from build123d import *

# Parameters (mm, degrees)
CROQUIS2_R              = 19
SALIENTE_EXTRUIR1_DEPTH = 7
CROQUIS2_4_R            = 6
SALIENTE_EXTRUIR2_DEPTH = 8
CROQUIS2_5_R            = 2
CORTAR_EXTRUIR2_DEPTH   = 8
CROQUIS5_R              = 3
CORTAR_EXTRUIR3_DEPTH   = 2


with BuildPart() as part:
    # Croquis2 → Saliente-Extruir1 (new body)
    with BuildSketch(Plane(origin=(0, 0, 0), x_dir=(1, 0, 0), z_dir=(0, 1, 0))):
        Circle(CROQUIS2_R)
    extrude(amount=SALIENTE_EXTRUIR1_DEPTH)

    # Croquis2<4> → Saliente-Extruir2 (add)
    with BuildSketch(Plane(origin=(0, 0, 0), x_dir=(1, 0, 0), z_dir=(0, 1, 0))):
        Circle(CROQUIS2_4_R)
    extrude(amount=-SALIENTE_EXTRUIR2_DEPTH)

    # Croquis2<5> → Cortar-Extruir2 (cut, through all)
    with BuildSketch(Plane(origin=(0, 0, 0), x_dir=(1, 0, 0), z_dir=(0, 1, 0))):
        with Locations((-15, 0)):
            Circle(CROQUIS2_5_R)
    extrude(amount=CORTAR_EXTRUIR2_DEPTH, mode=Mode.SUBTRACT)

    # Croquis5 → Cortar-Extruir3 (cut)
    with BuildSketch(Plane(origin=(0, 7, 0), x_dir=(1, 0, 0), z_dir=(0, 1, 0))):
        with Locations((-15, 0)):
            Circle(CROQUIS5_R)
    extrude(amount=-CORTAR_EXTRUIR3_DEPTH, mode=Mode.SUBTRACT)


solid = part.part
Design review of the part built by this model. Coordinates are the model's own, in mm. A direction names the side the tool comes from. Round coordinates to 2 decimals unless told otherwise and drop trailing zeros. Loops run counter-clockwise (first coordinate to the right, second up) from the corner with the lowest first, then second, coordinate; pieces in that order, holes last. Notation, with made-up numbers: (49, 40.5) - (102, 40.5) arc R34 ccw to (102, 77.5) - close; hole circle Ø9 at (68, 76.25). An arc over 180 degrees is marked (long way). One line per item, written item: value. Start each with the question number.
1) Consider section A-A on z = 0. Give the boundary of the cut face in (x, y), then the cut area to 3 significant figures.
2) To check wall thickness, follow L1, parallel to X at y = 2.15, z = 0; L2, parallel to X at y = 5.7, z = 0; L3, parallel to Y at x = 17, z = 6. State the ranges of each line that lie inside material, in increasing order. Write a range as from..to.
3) Consider section C-C on x = -15. Give the boundary of the cut face in (y, z), then the cut area to 3 significant figures.
4) Insertion check: pin 1 Ø4 at (x, z) = (-15, 14) entering from +Y; pin 2 Ø1.5 at (x, y) = (-13, 5) entering from -Z; pin 3 Ø8 at (x, y) = (3, -6.5) entering from -Z; pin 4 Ø4 at (y, z) = (2, 4) entering from +X. Each pin has a flat end and moves straight along its axis. Give the tip position at first contact, or say it passes through.
5) Consider section D-D on y = 3.5. Give the boundary of the cut face in (x, z), then the cut area to 3 significant figures.
6) Consider section B-B on x = 0. Give the boundary of the cut face in (y, z), then the cut area to 3 significant figures.
7) Draft analysis for pull direction X (two halves, no side actions). For faces 4 (the cylindrical face through (-18, 6, 0)), 5 (the cylindrical face through (8.767, 3.451, 16.856)), 6 (the flat face through (-4.5, 0, -4.5)), state which applies: +X half, -X half, draft (parallel to the pull), parting line (faces both ways), or undercut.
8) For faces 1 (the flat face through (-13, 5, 1)), 2 (the flat face through (0, -8, 0)), 3 (the cylindrical face through (-6, -4, 0)), list the 3-axis set-ups (+Z, -Z, +X, -X, +Y, -Y) from which the entire face can be reached by the end or side of a thin tool; tool diameter is ignored.
Reported:
1. outline: (-19, 0) - (-17, 0) - (-17, 5) - (-18, 5) - (-18, 7) - (-19, 7) - close; (-13, 0) - (-6, 0) - (-6, -8) - (6, -8) - (6, 0) - (19, 0) - (19, 7) - (-12, 7) - (-12, 5) - (-13, 5) - close
1. area: 330 mm^2
2. L1: x = -19..-17, -13..19
2. L2: x = -19..-18, -12..19
2. L3: y = 0..7
3. outline: (0, -11.66) - (7, -11.66) - (7, -3) - (5, -3) - (5, -2) - (0, -2) - close; (0, 2) - (5, 2) - (5, 3) - (7, 3) - (7, 11.66) - (0, 11.66) - close
3. area: 131 mm^2
4. pin 1: stops at y = 7
4. pin 2: stops at z = -14.52
4. pin 3: stops at z = -6
4. pin 4: stops at x = 18.89
5. outline: circle Ø38 at (0, 0); hole circle Ø4 at (-15, 0)
5. area: 1,120 mm^2
6. outline: (-8, -6) - (0, -6) - (0, -19) - (7, -19) - (7, 19) - (0, 19) - (0, 6) - (-8, 6) - close
6. area: 362 mm^2
7. face 4: undercut
7. face 5: parting line
7. face 6: draft
8. face 1: +Y
8. face 2: +Z, -Z, +X, -X, -Y
8. face 3: -Y
